from build123d import *

# Parameters (mm, degrees)
SKETCH_1_W          = 40
SKETCH_1_H          = 15
EXTRUDE_1_DEPTH     = 1.5
SKETCH_2_R          = 12
EXTRUDE_2_DEPTH     = 8
SKETCH_3_R          = 7
SKETCH_3_R_2        = 5
CUT_EXTRUDE_1_DEPTH = 3
SKETCH_4_R          = 5
CUT_EXTRUDE_2_DEPTH = 4.5
SKETCH_5_R          = 4
EXTRUDE_3_DEPTH     = 0.5
FILLET_3_R          = 1
FILLET_5_R          = 0.5
SKETCH_6_W          = 15
SKETCH_6_H          = 1.5
CUT_EXTRUDE_3_DEPTH = 41
FILLET_6_R          = 1
SKETCH_7_W          = 5
SKETCH_7_H          = 5
CUT_EXTRUDE_4_DEPTH = 1.5


with BuildPart() as part:
    # 草图1 → 凸台-拉伸1 (new body)
    with BuildSketch(Plane(origin=(0, 0, 0), x_dir=(1, 0, 0), z_dir=(0, 1, 0))):
        Rectangle(SKETCH_1_W, SKETCH_1_H)
    extrude(amount=EXTRUDE_1_DEPTH)

    # 草图2 → 凸台-拉伸2 (add)
    with BuildSketch(Plane(origin=(0, 1.5, 0), x_dir=(1, 0, 0), z_dir=(0, 1, 0))):
        Circle(SKETCH_2_R)
    extrude(amount=EXTRUDE_2_DEPTH)

    # 草图3 → 切除-拉伸1 (cut)
    with BuildSketch(Plane(origin=(0, 9.5, 0), x_dir=(1, 0, 0), z_dir=(0, 1, 0))):
        Circle(SKETCH_3_R)
        Circle(SKETCH_3_R_2, mode=Mode.SUBTRACT)
    extrude(amount=-CUT_EXTRUDE_1_DEPTH, mode=Mode.SUBTRACT)

    # 草图4 → 切除-拉伸2 (cut)
    with BuildSketch(Plane(origin=(0, 9.5, 0), x_dir=(1, 0, 0), z_dir=(0, 1, 0))):
        Circle(SKETCH_4_R)
    extrude(amount=-CUT_EXTRUDE_2_DEPTH, mode=Mode.SUBTRACT)

    # 草图5 → 凸台-拉伸3 (add)
    with BuildSketch(Plane(origin=(0, 5, 0), x_dir=(1, 0, 0), z_dir=(0, 1, 0))):
        Circle(SKETCH_5_R)
    extrude(amount=EXTRUDE_3_DEPTH)

    # 圆角3
    fillet_3_edges = [part.edges().sort_by_distance(p)[0] for p in [
        (-12, 9.5, 0),
        (-7, 9.5, 0),
    ]]
    fillet(fillet_3_edges, radius=FILLET_3_R)

    # 圆角5
    fillet_5_edges = [part.edges().sort_by_distance(p)[0] for p in [
        (-5, 6.5, 0),
    ]]
    fillet(fillet_5_edges, radius=FILLET_5_R)

    # 草图6 → 切除-拉伸3 (cut, through all)
    with BuildSketch(Plane(origin=(20, 0, 0), x_dir=(0, 0, -1), z_dir=(1, 0, 0))):
        with Locations((0, 0.75)):
            Rectangle(SKETCH_6_W, SKETCH_6_H)
    extrude(amount=-CUT_EXTRUDE_3_DEPTH, mode=Mode.SUBTRACT)

    # 圆角6
    fillet_6_edges = [part.edges().sort_by_distance(p)[0] for p in [
        (-12, 1.5, 0),
    ]]
    fillet(fillet_6_edges, radius=FILLET_6_R)

    # 草图7 → 切除-拉伸4 (cut)
    with BuildSketch(Plane.XZ.offset(-1.5)):
        Rectangle(SKETCH_7_W, SKETCH_7_H)
    extrude(amount=-CUT_EXTRUDE_4_DEPTH, mode=Mode.SUBTRACT)


solid = part.part
The listing builds one solid part. Answer for the finished solid, in the listing's coordinates (mm). A direction names the side the tool comes from. Give positions to 0.01 mm unless a question says otherwise; leave off trailing zeros. Write each loop counter-clockwise with the first axis right and the second up, starting at its lowest first coordinate (ties: lowest second). Pieces come first, ordered by that corner, then holes. Notation, with made-up numbers: (1, -34.5) -> (23, -34.5) arc R25 ccw to (23, -6.5) -> close; hole circle Ø11 at (38.5, 0.5). An arc over 180 degrees is marked (long way). One line per question, with ' | ' between items. Start each with the question number.
1. For a pull along Z with two mould halves and no side action, classify faces 4 (the flat face through (-4, 6.5, 4)), 5 (the flat face through (3, 1.5, 0)), 6 (the cylindrical face through (-11.99, 5.46, -0.53)) as pulls with the +Z half, pulls with the -Z half, needs draft (parallel to the pull), parting line crosses it, or undercut.
2. Find the intervals of material crossed by probe 1 along X at (y, z) = (5.25, 0); probe 2 along Z at (x, y) = (0, 5.7); probe 3 along Z at (x, y) = (0, 8.1), in increasing order.
3. Section A-A (x = 0) is taken. Determine the outline of the cut face in (y, z).
4. Given pin 1 Ø0.8 at (y, z) = (2.5, 1) entering from -X (3 decimals); pin 2 Ø4 at (x, z) = (1, 1) entering from +Y; pin 3 Ø1 at (y, z) = (5.5, -8) entering from +X, each flat-ended and moving along its own axis, determine where each tip first touches the part or whether it passes through.
5. For faces 1 (the flat face through (0, 5.5, 0)), 2 (the flat face through (-2, 9.5, 8)), 3 (the flat face through (-2.5, 2, 0)), determine the directions among +Z, -Z, +X, -X, +Y, -Y from which every point of the face is accessible in a straight line to the end or side of a thin tool.
6. Section C-C (y = 7.25) is taken. Determine the outline of the cut face in (x, z).
7. Section B-B (y = 3.5) is taken. Determine the outline of the cut face in (x, z), plus the area to 3 significant figures.
Response values:
1) face 4: undercut | face 5: needs draft | face 6: parting line crosses it
2) probe 1: -12 to -5, -4 to 4, 5 to 12 | probe 2: -12 to -5, 5 to 12 | probe 3: -12 to -7, 7 to 12
3) outline: (1.5, -11) arc R1 ccw to (2.5, -12) -> (8.5, -12) arc R1 ccw to (9.5, -11) -> (9.5, -8) arc R1 ccw to (8.5, -7) -> (6.5, -7) -> (6.5, -5.5) arc R0.5 ccw to (6, -5) -> (5, -5) -> (5, -4) -> (5.5, -4) -> (5.5, 4) -> (5, 4) -> (5, 5) -> (6, 5) arc R0.5 ccw to (6.5, 5.5) -> (6.5, 7) -> (8.5, 7) arc R1 ccw to (9.5, 8) -> (9.5, 11) arc R1 ccw to (8.5, 12) -> (2.5, 12) arc R1 ccw to (1.5, 11) -> (1.5, 2.5) -> (3, 2.5) -> (3, -2.5) -> (1.5, -2.5) -> close
4) pin 1: x = -11.985 | pin 2: y = 5.5 | pin 3: x = 9.37
5) face 1: +Y | face 2: +Z, -Z, +X, -X, +Y | face 3: -Y
6) outline: circle Ø24 at (0, 0); hole circle Ø14 at (0, 0)
7) outline: circle Ø24 at (0, 0) | area: 452 mm2
